Autodesk Inventor part; units mm, degrees
ref_plane "YZ Plane" through (0, 0, 0) normal (1, 0, 0) x (0, 1, 0)
ref_plane "XZ Plane" through (0, 0, 0) normal (0, 1, 0) x (-1, 0, 0)
ref_plane "XY Plane" through (0, 0, 0) normal (0, 0, 1) x (1, 0, 0)
sketch "스케치1" plane through (0, 0, 0) normal (1, 0, 0) x (0, 1, 0)
  line L0 (0, -41.5) -> (18, -41.5)
  line L1 (18, -41.5) -> (18, 59.6584) construction
  line L2 (0, 0) -> (0, -41.5)
  line L3 (84.3904, -3) -> (-15.1692, -3) construction
  arc A0 (63, -15) -> (75, -3) centre (63, -3) ccw
  line L4 (63, -15) -> (38, -15)
  line L5 (38, -15) -> (18, -41.5)
  line L6 (0, 35.5) -> (18, 35.5)
  line L7 (0, 0) -> (0, 35.5)
  arc A1 (75, -3) -> (63, 9) centre (63, -3) ccw
  line L8 (63, 9) -> (38, 9)
  line L9 (38, 9) -> (18, 35.5)
  dimension "d0" = 18
  dimension "d8" = 45
  dimension "d9" = 25
  dimension "d32" = 12
extrude "돌출1" add sketch "스케치1" along normal blind 6
sketch "스케치2" plane through (6, 0, 0) normal (1, 0, 0) x (0, 0, -1)
  line L0 (-58.8675, 4) -> (65.7315, 4) construction
  line L1 (-35.5, 0) -> (41.5, 0)
  circle A0 centre (31.5, 4) radius 1.75
  circle A1 centre (21.5, 4) radius 1.65
  line L2 (41.5, 0) -> (41.5, 18)
  line L3 (0, 13.8041) -> (0, -7.7982) construction
  circle A2 centre (-31.5, 4) radius 1.75
  circle A3 centre (-21.5, 4) radius 1.65
  point P0 (0, 0)
  dimension "d12" = 4
  dimension "d13" = 3.5
  dimension "d14" = 3.3
  dimension "d15" = 10
  dimension "d16" = 20
extrude "돌출2" cut sketch "스케치2" against normal blind 6
sketch "스케치4" plane through (6, 0, 0) normal (1, 0, 0) x (0, 0, -1)
  arc A0 (15, 63) -> (-9, 63) centre (3, 63) ccw
  circle A1 centre (3, 63) radius 6.5
  point P0 (0, 0)
  dimension "d25" = 13
extrude "돌출4" cut sketch "스케치4" against normal blind 4
sketch "스케치5" plane through (2, 63, -3) normal (1, 0, 0) x (0, 0, -1)
  circle A0 centre (0, 0) radius 4.85
  point P0 (-3, -63)
  dimension "d28" = 9.7
extrude "돌출5" cut sketch "스케치5" against normal blind 2
fillet "모깎기1" radius 1 1 edges at (6, 63, 3.5)
sketch "스케치6" plane through (0, 0, 0) normal (-1, 0, 0) x (0, 0, 1)
  line L0 (-41.5, 0) -> (-41.5, 18)
  line L1 (35.5, 0) -> (-41.5, 0)
  line L2 (-41.5, 18) -> (35.5, 18)
  line L3 (35.5, 18) -> (35.5, 0)
  line L4 (35.5, 0) -> (-41.5, 0)
  line L5 (-41.5, 0) -> (-41.5, 18)
  circle A0 centre (-31.5, 4) radius 1.75
  circle A1 centre (-31.5, 4) radius 1.75
  circle A2 centre (-21.5, 4) radius 1.65
  circle A3 centre (-21.5, 4) radius 1.65
  circle A4 centre (21.5, 4) radius 1.65
  circle A5 centre (21.5, 4) radius 1.65
  circle A6 centre (31.5, 4) radius 1.75
  circle A7 centre (31.5, 4) radius 1.75
  point P0 (0, 0)
extrude "돌출6" add sketch "스케치6" along normal blind 3.5
properties part number "탑(옆면수정)"
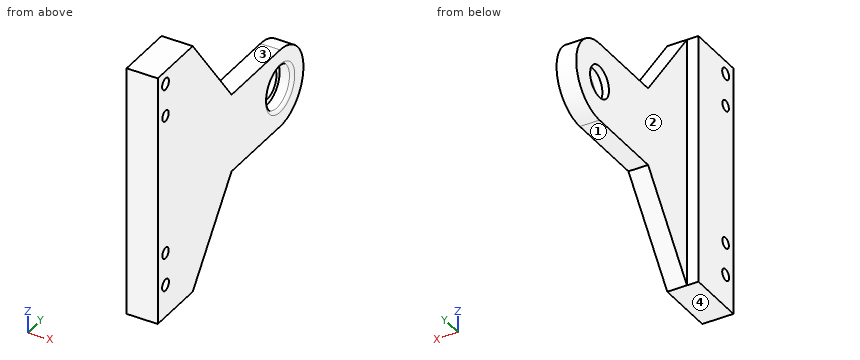
Here's how the part is built. I have some questions about the finished solid (model axes, mm). Face numbers are marked on the shaded views. A direction names the side the tool comes from. Coordinates: 2 decimals unless noted, no trailing zeros. Order: outer loops, then holes, each group sorted by start corner. A loop starts at its lowest first (then second) coordinate and runs counter-clockwise, first axis right, second up.
1) Imagine slicing it at B-B on z = -3. List the corners of the cut face in (x, y) for me.
2) I need wall thicknesses on line 1 (Z direction, x = 1.8, y = 4); line 2 (Y direction, x = -1.6, z = -31.5); line 3 (Y direction, x = 3.2, z = -3). Which ranges of each line are inside material? Lowest first, please.
3) Imagine slicing it at D-D on y = 48.5. List the corners of the cut face in (x, z) for me.
4) Will these pins go through, and if not, where does the flat tip stop? pin 1 (4 mm diameter, centred on x = -1.5, y = 46.5, fed in from -Z); pin 2 (3 mm diameter, centred on y = 4, z = -21.5, fed in from +X) (1 decimal); pin 3 (2 mm diameter, centred on y = 50.5, z = -9, fed in from -X); pin 4 (1.8 mm diameter, centred on x = -1, z = 11, fed in from +Y).
5) Which directions (+Z, -Z, +X, -X, +Y, -Y) give clear straight access to the entire face, cutting with the end or side of a thin tool? Please do the marked faces 1, 2, 3 and 4.
6) Imagine slicing it at A-A on x = 1. List the corners of the cut face in (y, z) for me, and give its area (3 significant figures).
7) Imagine slicing it at C-C on y = 4. List the corners of the cut face in (x, z) for me.
Response values:
1. outline: (-3.5, 0) - (6, 0) - (6, 55.5) arc R1 ccw to (5, 56.5) - (2, 56.5) - (2, 58.15) - (0, 58.15) - (0, 18) - (-3.5, 18) - close; (0, 67.85) - (2, 67.85) - (2, 69.5) - (5, 69.5) arc R1 ccw to (6, 70.5) - (6, 75) - (0, 75) - close
2. line 1: z = -41.5 to -33.25, -29.75 to -23.15, -19.85 to 19.85, 23.15 to 29.75, 33.25 to 35.5
2. line 2: y = 0 to 2.25, 5.75 to 18
2. line 3: y = 0 to 56.5, 69.5 to 75
3. outline: (0, -15) - (6, -15) - (6, 9) - (0, 9) - close
4. pin 1: stops at z = -15
4. pin 2: passes through
4. pin 3: stops at x = 0
4. pin 4: stops at y = 18
5. face 1: -Z, +X, -X, +Y
5. face 2: +Z, -Z, -X, +Y
5. face 3: +Z, +X, -X, +Y
5. face 4: -Z, +X, -X, +Y, -Y
6. outline: (0, -41.5) - (18, -41.5) - (38, -15) - (63, -15) arc R12 ccw to (63, 9) - (38, 9) - (18, 35.5) - (0, 35.5) - close; hole circle Ø3.5 at (4, -31.5); hole circle Ø3.5 at (4, 31.5); hole circle Ø3.3 at (4, -21.5); hole circle Ø3.3 at (4, 21.5); hole circle Ø9.7 at (63, -3)
6. area: 3,110 mm2
7. outline: (-3.5, -41.5) - (6, -41.5) - (6, -33.25) - (-3.5, -33.25) - close; (-3.5, -29.75) - (6, -29.75) - (6, -23.15) - (-3.5, -23.15) - close; (-3.5, -19.85) - (6, -19.85) - (6, 19.85) - (-3.5, 19.85) - close; (-3.5, 23.15) - (6, 23.15) - (6, 29.75) - (-3.5, 29.75) - close; (-3.5, 33.25) - (6, 33.25) - (6, 35.5) - (-3.5, 35.5) - close
